Study the drawing (mm; zero at the part's minimum x, y, z) and answer. A direction names the side the tool comes from. Coordinates: 2 decimals unless noted, no trailing zeros. Loops run counter-clockwise (first coordinate to the right, second up) from the corner with the lowest first, then second, coordinate; pieces in that order, holes last.
Q1. Section B-B (z = 260) is taken. Give the vertices of the cut face in (x, y).
Q2. Section C-C (y = 58.5) is taken. Give the vertices of the cut face in (x, z), then the cut area to 3 significant figures.
Q3. Which of the six approach directions +Z, -Z, +X, -X, +Y, -Y give full straight-line access (tool end or side, diameter ignored) to the marked faces 1, 2 and 3?
Q4. Flat-ended cylindrical pins translate along their axes: P1, Ø15, axis at x = 23.5, z = 290.5, coming from the +Y side; P2, Ø20.5, axis at x = 36.5, y = 70.5, coming from the -Z side. Find the tip coordinate at first contact, or state that the pin passes through.
Q5. Straight lines are drawn through the part: line 1 (Z direction, x = 11, y = 71); line 2 (Y direction, x = 43.5, z = 87). For each, find the intervals that lie inside material, in ascending order.
Q6. Section A-A (x = 38) is taken. Give the vertices of the cut face in (y, z).
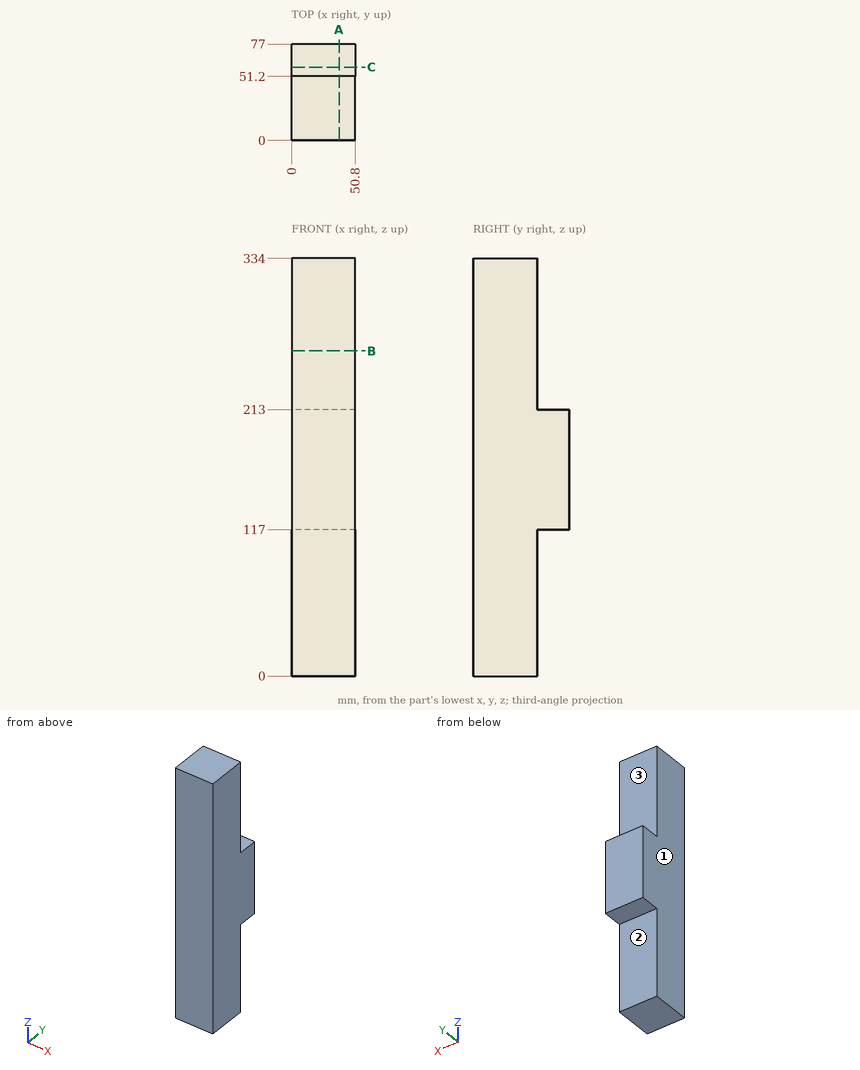
Numbers:
1. outline: (0, 0) - (50.8, 0) - (50.8, 51.2) - (0, 51.2) - close
2. outline: (0, 117) - (50.8, 117) - (50.8, 213) - (0, 213) - close
2. area: 4,880 mm2
3. face 1: +Z, -Z, -X, +Y, -Y
3. face 2: -Z, +X, -X, +Y
3. face 3: +Z, +X, -X, +Y
4. P1: stops at y = 51.2
4. P2: stops at z = 117
5. line 1: z = 117 to 213
5. line 2: y = 0 to 51.2
6. outline: (0, 0) - (51.2, 0) - (51.2, 117) - (77, 117) - (77, 213) - (51.2, 213) - (51.2, 334) - (0, 334) - close
